Source: three-view drawing plus pictorial views. Frame: mm from the lowest corner of the part. Round coordinates to 2 decimals unless told otherwise and drop trailing zeros. Order: outer loops, then holes, each group sorted by start corner. A loop starts at its lowest first (then second) coordinate and runs counter-clockwise, first axis right, second up. Notation, with made-up numbers: (4, 76) -> (36, 76) arc R20 ccw to (36, 98) -> close; hole circle Ø1 at (24.25, -27). An arc over 180 degrees is marked (long way). Answer as CSV lines item,"result".
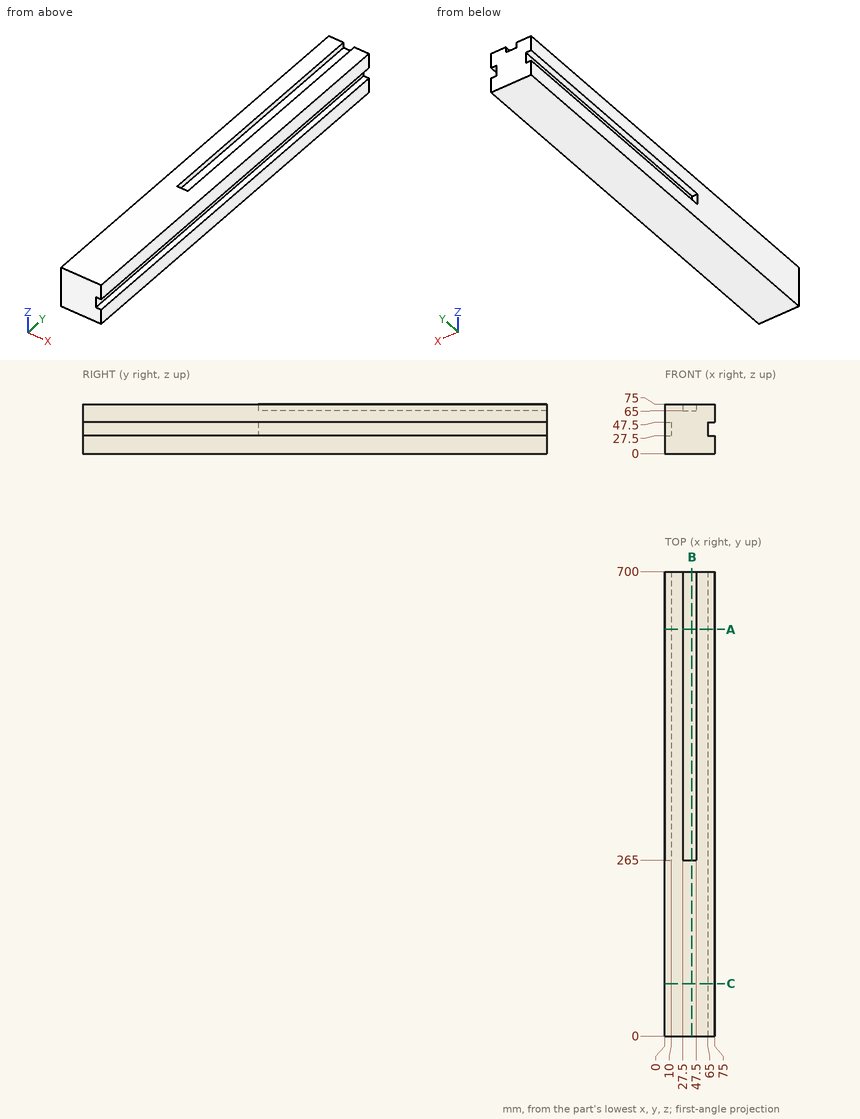
1. Section query C-C on y = 79. Return loops of the section in (x, z).
Results below:
outline,"(0, 0) -> (75, 0) -> (75, 27.5) -> (65, 27.5) -> (65, 47.5) -> (75, 47.5) -> (75, 75) -> (0, 75) -> close"
2. Section query A-A on y = 613. Return loops of the section in (x, z).
Results below:
outline,"(0, 0) -> (75, 0) -> (75, 27.5) -> (65, 27.5) -> (65, 47.5) -> (75, 47.5) -> (75, 75) -> (47.5, 75) -> (47.5, 65) -> (27.5, 65) -> (27.5, 75) -> (0, 75) -> (0, 47.5) -> (10, 47.5) -> (10, 27.5) -> (0, 27.5) -> close"
3. Line query: L1, parallel to Z at x = 7, y = 324; L2, parallel to Z at x = 43, y = 630. Output: solid intervals per line, ascending. Write a range as [from, to].
Results below:
L1,"[0, 27.5], [47.5, 75]"
L2,"[0, 65]"
4. Pin query (flat end, axial travel): pin 1 (16 mm diameter, centred on x = 38, y = 543.5, fed in from +Z); pin 2 (8 mm diameter, centred on x = 4.5, z = 36, fed in from +Y). Return the tip coordinate at first contact, or that it passes through.
Results below:
pin 1,"z = 65"
pin 2,"y = 265"
5. Section query B-B on x = 41. Return loops of the section in (y, z).
Results below:
outline,"(0, 0) -> (700, 0) -> (700, 65) -> (265, 65) -> (265, 75) -> (0, 75) -> close"
